Could you check a few things on this drawing? It's one solid part, dimensions in mm from its lowest x, y, z. Give positions to 0.01 mm unless a question says otherwise; leave off trailing zeros. Loops run counter-clockwise (first coordinate to the right, second up) from the corner with the lowest first, then second, coordinate; pieces in that order, holes last. Notation, with made-up numbers: (-20.75, -32) - (2.25, -32) arc R26 ccw to (2.25, 6) - close; hole circle Ø11 at (-2, 83.5). An arc over 180 degrees is marked (long way). Return JSON: item names as keys, results as strings. Group by question number.
(1) If we mould it in two halves opening along Y, with no side actions, what happens to the marked faces 1 and 2? For each: released by +Y, released by -Y, zero draft, split by the parting line, or undercut.
(2) If we section it at B-B (x = 9.35): Please give me the cut outline in (y, z).
(3) I need wall thicknesses on probe 1 along X at (y, z) = (3.4, 9.35); probe 2 along X at (y, z) = (4.6, 9.35); probe 3 along Y at (x, z) = (6, 1.75). Which ranges of each line are inside material? Lowest first, please. Write a range as [from, to].
(4) If we section it at C-C (y = 3.15): Please give me the cut outline in (x, z), then the cut area to 3 significant figures.
(5) For P1, Ø5, axis at x = 15, z = 12, coming from the +Y side; P2, Ø8, axis at x = 5.5, z = 4.5, coming from the -Y side, each with a flat end and sliding along its axis, tell me the tip position at first contact or that it passes through.
(6) If we section it at A-A (z = 9.35): Please give me the cut outline in (x, y).
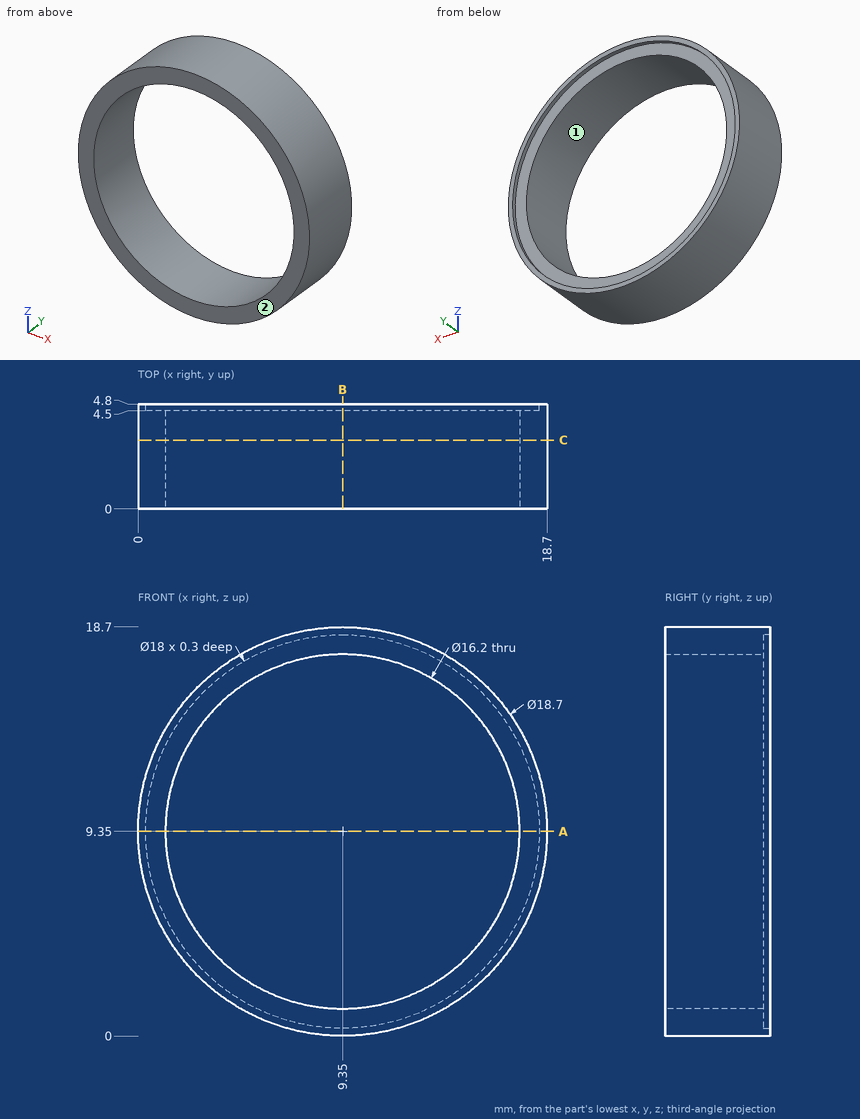
Values:
{
 "1": {"face 1": "zero draft", "face 2": "released by -Y"},
 "2": {"outline": "(0, 0) - (4.8, 0) - (4.8, 0.35) - (4.5, 0.35) - (4.5, 1.25) - (0, 1.25) - close; (0, 17.45) - (4.5, 17.45) - (4.5, 18.35) - (4.8, 18.35) - (4.8, 18.7) - (0, 18.7) - close"},
 "3": {"probe 1": "[0, 1.25], [17.45, 18.7]", "probe 2": "[0, 0.35], [18.35, 18.7]", "probe 3": "[0, 4.5]"},
 "4": {"outline": "circle Ø18.7 at (9.35, 9.35); hole circle Ø16.2 at (9.35, 9.35)", "area": "68.5 mm2"},
 "5": {"P1": "y = 4.5", "P2": "y = 0"},
 "6": {"outline": "(0, 0) - (1.25, 0) - (1.25, 4.5) - (0.35, 4.5) - (0.35, 4.8) - (0, 4.8) - close; (17.45, 0) - (18.7, 0) - (18.7, 4.8) - (18.35, 4.8) - (18.35, 4.5) - (17.45, 4.5) - close"}
}
